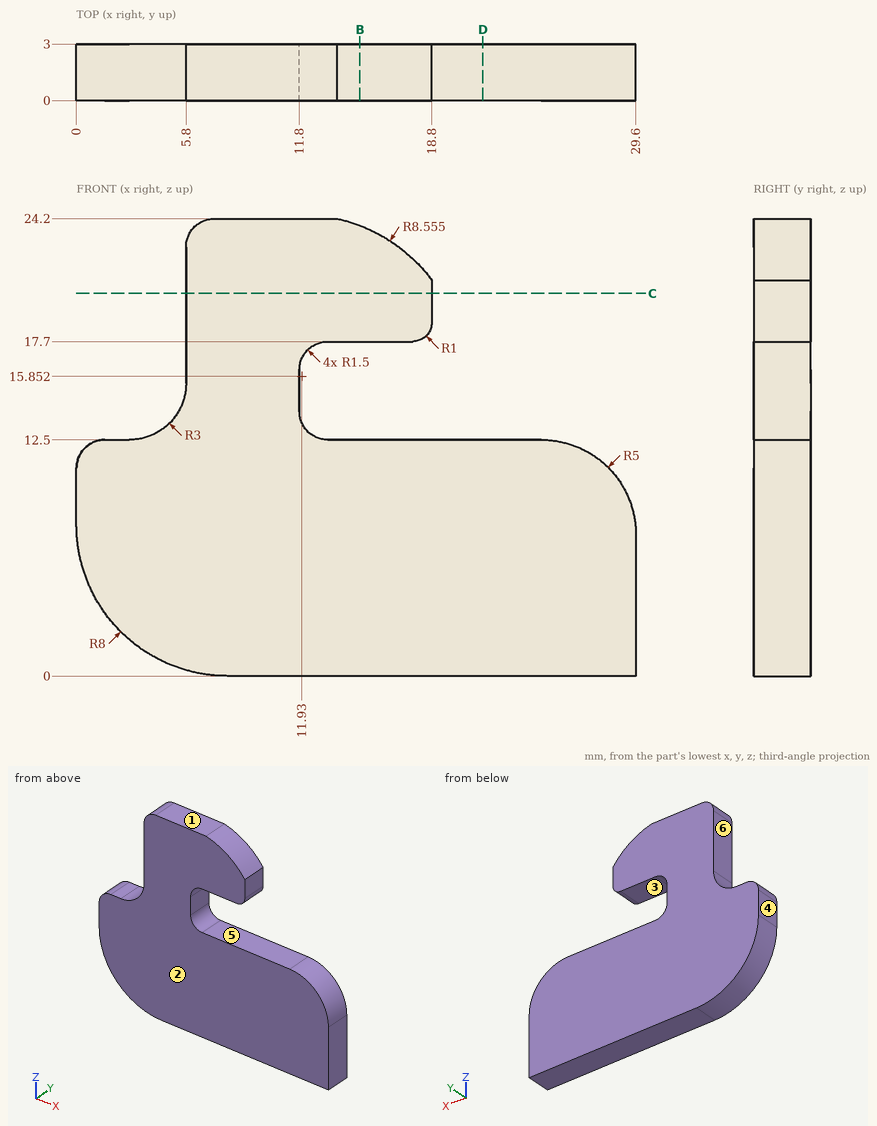
Here's the drawing with two shaded views (mm, measured from the low corner). I have some questions. A direction names the side the tool comes from. Coordinates: 2 decimals unless noted, no trailing zeros. Write each loop counter-clockwise with the first axis right and the second up, starting at its lowest first coordinate (ties: lowest second). Pieces come first, ordered by that corner, then holes. Notation, with made-up numbers: (-2, 79.5) -> (41, 79.5) arc R9 cw to (41, 83.5) -> close; hole circle Ø3 at (-8.5, 24). An arc over 180 degrees is marked (long way). Write item = value, one per line. Start each with the question number.
(1) I want a section at C-C (z = 20.25). Please give me the cut outline in (x, y).
(2) I want a section at B-B (x = 15). Please give me the cut outline in (y, z).
(3) Which directions (+Z, -Z, +X, -X, +Y, -Y) give clear straight access to the entire face, cutting with the end or side of a thin tool? Please do the marked faces 4, 5 and 6.
(4) Will these pins go through, and if not, where does the flat tip stop? pin 1 (1 mm diameter, centred on x = 25.5, y = 1, fed in from +Z); pin 2 (0.7 mm diameter, centred on y = 2, z = 15.5, fed in from +X).
(5) We'd pull the mould along Z, two halves only. Please class the marked faces 1, 2 and 3: released by +Z, released by -Z, zero draft, split by the parting line, or undercut.
(6) I want a section at D-D (x = 21.5). Please give me the cut outline in (y, z), plus the area to 3 significant figures.
(7) I need wall thicknesses on line 1 (Z direction, x = 13.5, y = 2.65); line 2 (Z direction, x = 24.25, y = 1.5); line 3 (Z direction, x = 15.5, y = 2.6). Which ranges of each line are inside material? Lowest first, please. Write a range as [from, to].
Result set:
q1.outline = (5.8, 0) -> (18.8, 0) -> (18.8, 3) -> (5.8, 3) -> close
q2.outline = (0, 0) -> (3, 0) -> (3, 12.5) -> (0, 12.5) -> close; (0, 17.7) -> (3, 17.7) -> (3, 23.84) -> (0, 23.84) -> close
q3.face_4 = +Z, -Z, -X, +Y, -Y
q3.face_5 = +X, +Y, -Y
q3.face_6 = +Z, -X, +Y, -Y
q4.pin_1 = 12.48
q4.pin_2 = 11.8
q5.face_1 = released by +Z
q5.face_2 = zero draft
q5.face_3 = undercut
q6.outline = (0, 0) -> (3, 0) -> (3, 12.5) -> (0, 12.5) -> close
q6.area = 37.5 mm2
q7.line_1 = [0, 12.5], [17.7, 24.2]
q7.line_2 = [0, 12.5]
q7.line_3 = [0, 12.5], [17.7, 23.63]
